Geometry check sheet. Reference: the model listing, model coordinates, mm. A direction names the side the tool comes from. Give positions to 0.01 mm unless a question says otherwise; leave off trailing zeros. Loops run counter-clockwise (first coordinate to the right, second up) from the corner with the lowest first, then second, coordinate; pieces in that order, holes last. Notation, with made-up numbers: (55, 62) -> (105, 62) arc R27 ccw to (105, 79) -> close; hole circle Ø2 at (-33, 50.25). An arc over 180 degrees is marked (long way). One line per item, written item: value. Start each with the question number.
(1) Gauge pin test, flat ends, axial feed: pin 1 Ø1.5 at (x, y) = (-2.5, 3) entering from -Z; pin 2 Ø1 at (x, z) = (1, -0.5) entering from +Y; pin 3 Ø5.5 at (x, y) = (0, 0) entering from -Z. Record the tip position at first contact, or that the pin passes through.
(2) Sectioned sample at C-C, the plane z = 1.15. Record the cut outline in (x, y), then the cut area to 3 significant figures.
(3) Scan lines: line 1 along Y through (x, z) = (0, 1.45); line 2 along Y through (x, z) = (0, -1.4); line 3 along Z through (x, y) = (-4, -0.5). Record each from-to range of solid material in increasing order. Write a range as from..to.
(4) Tool access check on faces 4 (the face through (-1.08, -4.88, 0.32)), 5 (the face through (-3, 0, 0)), 6 (the face through (2, 3, -1.3)). Record the directions out of +Z, -Z, +X, -X, +Y, -Y that give a thin tool (end or side, any length) a straight path to the whole face; none if there is none.
(5) Draft check along Y on faces 1 (the face through (2, 3, 1.3)), 2 (the face through (5.595, 0.246, -1.204)), 3 (the face through (2, 5, -0.9)). Enter one of: pulls with the +Y half, pulls with the -Y half, needs draft (parallel to the pull), parting line crosses it, or undercut.
(6) Sectioned sample at A-A, the plane y = 0. Record the cut outline in (x, z).
from build123d import *

# Parameters (mm, degrees)
SKETCH_1_R          = 5
EXTRUDE_1_DEPTH     = 1.5
SKETCH_4_R          = 5.6
EXTRUDE_2_DEPTH     = 0.6
SKETCH_2_R          = 3
CUT_EXTRUDE_1_DEPTH = 4
SKETCH_3_R          = 4.5
SKETCH_3_R_2        = 3.3
CUT_EXTRUDE_2_DEPTH = 0.2


with BuildPart() as part:
    # 草圖1 → 填料-伸長1 (new body, symmetric)
    with BuildSketch(Plane.XY):
        Circle(SKETCH_1_R)
    extrude(amount=EXTRUDE_1_DEPTH, both=True)

    # 草圖4 → 填料-伸長2 (add)
    with BuildSketch(Plane(origin=(0, 0, -1.5), x_dir=(-1, 0, 0), z_dir=(0, 0, -1))):
        Circle(SKETCH_4_R)
    extrude(amount=-EXTRUDE_2_DEPTH)

    # 草圖2 → 除料-伸長1 (cut, through all)
    with BuildSketch(Plane.XY.offset(1.5)):
        Circle(SKETCH_2_R)
    extrude(amount=-CUT_EXTRUDE_1_DEPTH, mode=Mode.SUBTRACT)

    # 草圖3 → 除料-伸長2 (cut)
    with BuildSketch(Plane.XY.offset(1.5)):
        Circle(SKETCH_3_R)
        Circle(SKETCH_3_R_2, mode=Mode.SUBTRACT)
    cut_extrude_2 = extrude(amount=-CUT_EXTRUDE_2_DEPTH, mode=Mode.SUBTRACT)

    # 鏡射1: 除料-伸長2 across plane
    add(cut_extrude_2.mirror(Plane.XY), mode=Mode.SUBTRACT)


solid = part.part
Calculated:
1. pin 1: stops at z = -1.5
1. pin 2: stops at y = 5.56
1. pin 3: passes through
2. outline: circle Ø10 at (0, 0); hole circle Ø6 at (0, 0)
2. area: 50.3 mm2
3. line 1: y = -5..-4.5, -3.3..-3, 3..3.3, 4.5..5
3. line 2: y = -5.6..-4.5, -3.3..-3, 3..3.3, 4.5..5.6
3. line 3: z = -1.3..1.3
4. face 4: +Z
4. face 5: +Z, -Z
4. face 6: -Z
5. face 1: undercut
5. face 2: parting line crosses it
5. face 3: needs draft
6. outline: (-5.6, -1.5) -> (-4.5, -1.5) -> (-4.5, -1.3) -> (-3.3, -1.3) -> (-3.3, -1.5) -> (-3, -1.5) -> (-3, 1.5) -> (-3.3, 1.5) -> (-3.3, 1.3) -> (-4.5, 1.3) -> (-4.5, 1.5) -> (-5, 1.5) -> (-5, -0.9) -> (-5.6, -0.9) -> close; (3, -1.5) -> (3.3, -1.5) -> (3.3, -1.3) -> (4.5, -1.3) -> (4.5, -1.5) -> (5.6, -1.5) -> (5.6, -0.9) -> (5, -0.9) -> (5, 1.5) -> (4.5, 1.5) -> (4.5, 1.3) -> (3.3, 1.3) -> (3.3, 1.5) -> (3, 1.5) -> close
